Input: part model. Units: mm. Frame: model coordinates. A direction names the side the tool comes from. Coordinates: 2 decimals unless noted, no trailing zeros. Order: outer loops, then holes, each group sorted by start corner. A loop starts at its lowest first (then second) coordinate and runs counter-clockwise, first axis right, second up. Notation, with made-up numbers: (31.25, 63) - (55.25, 63) arc R17 ccw to (55.25, 92) - close; hole circle Ø3 at (82, 5.5). An arc over 180 degrees is marked (long way). Answer as CSV lines item,"result". Start each with the question number.
Item 1: Material intervals for line 1 along Z through (x, y) = (0.5, 22.5); line 2 along Z through (x, y) = (3.25, -6.5); line 3 along Y through (x, z) = (-0.5, 2.75), sorted ascending.
Item 2: Access query for faces 5 (the flat face through (0, -4.5, 0)), 6 (the flat face through (-5, -1, 0)). Directions: +Z, -Z, +X, -X, +Y, -Y. A direction counts if a zero-diameter tool reaches every point of the face in a straight line with its end or side. Return the directions, or none.
Item 3: Section D-D (y = -22.5). Output: boundary loops of the cut face in (x, z).
Item 4: Section B-B (z = 0). Output: boundary loops of the cut face in (x, y), and give its area (3 significant figures).
Item 5: Section A-A (y = -6.5). Output: boundary loops of the cut face in (x, z), and give its area (3 significant figures).
Item 6: Section C-C (x = -0.25). Output: boundary loops of the cut face in (y, z), and give its area (3 significant figures).
Item 7: Draft query along Y for faces 1 (the flat face through (0, -9.5, 0)), 2 (the flat face through (0, 1, -14.226)), 3 (the flat face through (0, -7, -5.5)), 4 (the flat face through (0, 42.852, 0)). Return one class per face: +Y half, -Y half, draft (parallel to the pull), parting line (faces both ways), or undercut.
Autodesk Inventor part; units mm, degrees
ref_plane "UpperRodPlane" through (0, 22.5, 0) normal (0, 1, 0) x (-1, 0, 0)
ref_plane "LowerRodPlane" through (0, -22.5, 0) normal (0, 1, 0) x (-1, 0, 0)
ref_plane "RearClearancePlane" through (0, 0, -11) normal (0, 0, 1) x (1, 0, 0)
sketch "Sketch1" plane through (0, 0, 0) normal (1, 0, 0) x (0, 1, 0)
  circle A0 centre (22.5, 0) radius 9.5
  circle A1 centre (-22.5, 0) radius 9.5
  line L0 (-4.5, 5.5) -> (-9.5, 5.5)
  line L1 (-9.5, 5.5) -> (-9.5, -5.5)
  line L2 (-9.5, -5.5) -> (-4.5, -5.5)
  line L3 (-4.5, -5.5) -> (-4.5, 5.5)
  line L4 (-4.5, 5.5) -> (-9.5, -5.5) construction
  line L5 (-9.5, 5.5) -> (-4.5, -5.5) construction
  line L6 (42.8516, -14.2259) -> (-42.8516, -14.2259)
  line L7 (-42.8516, -14.2259) -> (-42.8516, 14.2259)
  line L8 (-42.8516, 14.2259) -> (42.8516, 14.2259)
  line L9 (42.8516, 14.2259) -> (42.8516, -14.2259)
  line L10 (42.8516, -14.2259) -> (-42.8516, 14.2259) construction
  line L11 (-42.8516, -14.2259) -> (42.8516, 14.2259) construction
  point P0 (0, 0)
  point P1 (-7, 0)
  dimension "d3" = 19
  dimension "d4" = 19
  dimension "d5" = 11
  dimension "d6" = 13
  dimension "d7" = 27
extrude "Extrusion1" add sketch "Sketch1" along normal mid plane 10
properties part number "E-Axis v2.0"
Determined:
1,line 1,"z = -14.23 to -9.5, 9.5 to 14.23"
1,line 2,"z = -14.23 to -5.5, 5.5 to 14.23"
1,line 3,"y = -42.85 to -31.59, -13.41 to -9.5, -4.5 to 13.41, 31.59 to 42.85"
2,face 5,"+X, -X"
2,face 6,"+Z, -Z, -X, +Y, -Y"
3,outline,"(-5, -14.23) - (5, -14.23) - (5, -9.5) - (-5, -9.5) - close; (-5, 9.5) - (5, 9.5) - (5, 14.23) - (-5, 14.23) - close"
4,outline,"(-5, -42.85) - (5, -42.85) - (5, -32) - (-5, -32) - close; (-5, -13) - (5, -13) - (5, -9.5) - (-5, -9.5) - close; (-5, -4.5) - (5, -4.5) - (5, 13) - (-5, 13) - close; (-5, 32) - (5, 32) - (5, 42.85) - (-5, 42.85) - close"
4,area,"427 mm^2"
5,outline,"(-5, -14.23) - (5, -14.23) - (5, -5.5) - (-5, -5.5) - close; (-5, 5.5) - (5, 5.5) - (5, 14.23) - (-5, 14.23) - close"
5,area,"175 mm^2"
6,outline,"(-42.85, -14.23) - (42.85, -14.23) - (42.85, 14.23) - (-42.85, 14.23) - close; hole circle Ø19 at (-22.5, 0); hole (-9.5, -5.5) - (-4.5, -5.5) - (-4.5, 5.5) - (-9.5, 5.5) - close; hole circle Ø19 at (22.5, 0)"
6,area,"1,820 mm^2"
7,face 1,"undercut"
7,face 2,"draft"
7,face 3,"undercut"
7,face 4,"+Y half"
